Model file for the job. Use its own axes, mm. Face numbers are marked on the shaded views. Round coordinates to 2 decimals unless told otherwise and drop trailing zeros. Write each loop counter-clockwise with the first axis right and the second up, starting at its lowest first coordinate (ties: lowest second). Pieces come first, ordered by that corner, then holes. Notation, with made-up numbers: (70, 33.5) - (114, 33.5) arc R20 cw to (114, 59.5) - close; hole circle Ø3 at (46.5, 26). An arc over 180 degrees is marked (long way). One line per item, written item: value.
from build123d import *

# Parameters (mm, degrees)
SKETCH_1_R          = 9
EXTRUDE_1_DEPTH     = 113.684766057
EXTRUDE_START       = -113.684766057
EXTRUDE_3_OUTLINE_R = 33.917711518
EXTRUDE_3_DEPTH     = 113.684766057


# Read off the part's stored shape, not the designer's step: Вырез-Вытянуть3
with BuildPart() as part:
    # Эскиз1 → Бобышка-Вытянуть1 (new body)
    with BuildSketch(Plane.XY):
        with BuildLine():
            ThreePointArc((-50, -37.5), (-44.194173824, -44.194173824), (-37.5, -50))
            Line((-37.5, -50), (37.5, -50))
            ThreePointArc((37.5, -50), (44.194173824, -44.194173824), (50, -37.5))
            Line((50, -37.5), (50, 37.5))
            ThreePointArc((50, 37.5), (44.194173824, 44.194173824), (37.5, 50))
            Line((37.5, 50), (-37.5, 50))
            ThreePointArc((-37.5, 50), (-44.194173824, 44.194173824), (-50, 37.5))
            Line((-50, 37.5), (-50, -37.5))
        make_face()
        with Locations((-32.526911935, -32.526911935)):
            Circle(SKETCH_1_R, mode=Mode.SUBTRACT)
        with Locations((32.526911935, -32.526911935)):
            Circle(SKETCH_1_R, mode=Mode.SUBTRACT)
        with Locations((-32.526911935, 32.526911935)):
            Circle(SKETCH_1_R, mode=Mode.SUBTRACT)
        with Locations((32.526911935, 32.526911935)):
            Circle(SKETCH_1_R, mode=Mode.SUBTRACT)
    extrude(amount=EXTRUDE_1_DEPTH)

    # Вырез-Вытянуть3 outline → Вырез-Вытянуть3 (cut)
    with BuildSketch(Plane.XY.offset(113.684766057).offset(EXTRUDE_START)):
        Circle(EXTRUDE_3_OUTLINE_R)
    extrude(amount=EXTRUDE_3_DEPTH, mode=Mode.SUBTRACT)


solid = part.part
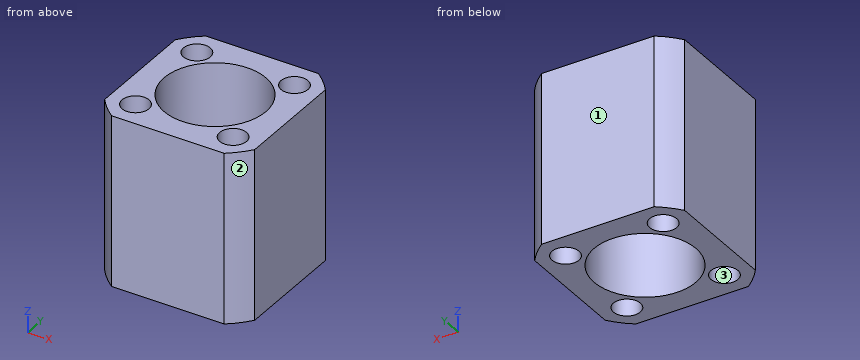
1. Drop a flat-ended pin along its axis: pin 1 (11 mm diameter, centred on x = -32.53, y = 32.53, fed in from +Z). Give the stop position or say it passes through.
Report:
pin 1: through
2. Band-saw the part on D-D on x = 40. Write the cut outline in (y, z), plus the area to 3 significant figures.
Report:
outline: (-48.02, 0) - (-37.54, 0) - (-37.54, 113.68) - (-48.02, 113.68) - close; (-27.51, 0) - (27.51, 0) - (27.51, 113.68) - (-27.51, 113.68) - close; (37.54, 0) - (48.02, 0) - (48.02, 113.68) - (37.54, 113.68) - close
area: 8,640 mm²
3. Band-saw the part on C-C on z = 82. Write the cut outline in (x, y), plus the area to 3 significant figures.
Report:
outline: (-50, -37.5) arc R62.5 ccw to (-37.5, -50) - (37.5, -50) arc R62.5 ccw to (50, -37.5) - (50, 37.5) arc R62.5 ccw to (37.5, 50) - (-37.5, 50) arc R62.5 ccw to (-50, 37.5) - close; hole circle Ø18 at (-32.53, -32.53); hole circle Ø18 at (-32.53, 32.53); hole circle Ø67.84 at (0, 0); hole circle Ø18 at (32.53, -32.53); hole circle Ø18 at (32.53, 32.53)
area: 5,090 mm²
4. Mould opens along X. For the marked faces 1, 2 and 3 say: released by +X, released by -X, zero draft, split by the parting line, or undercut.
Report:
face 1: zero draft
face 2: released by +X
face 3: undercut
5. Band-saw the part on A-A on x = 0. Write the cut outline in (y, z), plus the area to 3 significant figures.
Report:
outline: (-50, 0) - (-33.92, 0) - (-33.92, 113.68) - (-50, 113.68) - close; (33.92, 0) - (50, 0) - (50, 113.68) - (33.92, 113.68) - close
area: 3,660 mm²
6. Wall check: probe 1 along X at (y, z) = (25.5, 83); probe 2 along Y at (x, z) = (29, 73); probe 3 along Y at (x, z) = (-1, 82). Give the ranges that are in metal, low to high. Write a range as [from, to].
Report:
probe 1: [-50, -38.15], [-26.9, -22.36], [22.36, 26.9], [38.15, 50]
probe 2: [-50, -40.81], [-24.25, -17.59], [17.59, 24.25], [40.81, 50]
probe 3: [-50, -33.9], [33.9, 50]
